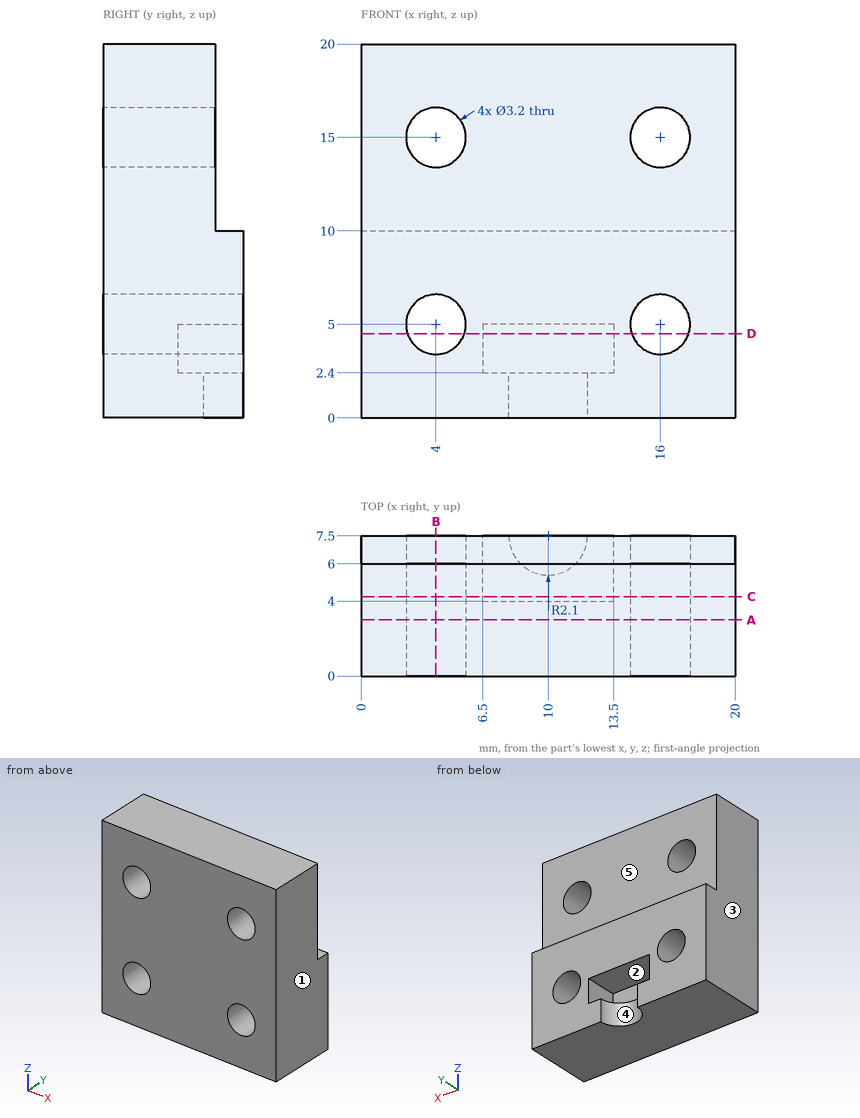
Here's the drawing with two shaded views (mm, measured from the low corner). I have some questions. A direction names the side the tool comes from. Coordinates: 2 decimals unless noted, no trailing zeros. Write each loop counter-clockwise with the first axis right and the second up, starting at its lowest first coordinate (ties: lowest second). Pieces come first, ordered by that corner, then holes. Notation, with made-up numbers: M 57.25,33.5 L 116.25,33.5 A32 ccw 116.25,59.5 Z; hole C 74,15.25 d2. An arc over 180 degrees is marked long. Answer as CSV lines item,"result". Start each with the question number.
1) For P1, Ø5, axis at x = 5.5, z = 14, coming from the +Y side; P2, Ø1.2, axis at x = 9.5, y = 7, coming from the +Z side; P3, Ø0.8, axis at x = 11.5, z = 3.5, coming from the +Y side, each with a flat end and sliding along its axis, tell me the tip position at first contact or that it passes through.
2) For the marked faces 1 and 2, which set-ups out of +Z, -Z, +X, -X, +Y, -Y let a thin tool reach every point of the face, with its end or its side?
3) We'd pull the mould along X, two halves only. Please class the marked faces 3, 4 and 5: +X half, -X half, draft (parallel to the pull), parting line (faces both ways), or undercut.
4) Please list where these lines run through material, in increasing order: line 1 (Z direction, x = 16, y = 2.75); line 2 (X direction, y = 3.4, z = 15); line 3 (X direction, y = 1, z = 15.5). Write a range as from..to.
5) I want a section at A-A, the plane y = 3. Please give me the cut outline in (x, z).
6) I want a section at D-D, the plane z = 4.5. Please give me the cut outline in (x, y), and give its area (3 significant figures).
7) I want a section at B-B, the plane x = 4. Please give me the cut outline in (y, z).
8) I want a section at C-C, the plane y = 4.25. Please give me the cut outline in (x, z), and give its area (3 significant figures).
Data:
1,P1,"stops at y = 6"
1,P2,"stops at z = 10"
1,P3,"stops at y = 4"
2,face 1,"+Z, -Z, +X, +Y, -Y"
2,face 2,"+Y"
3,face 3,"-X half"
3,face 4,"undercut"
3,face 5,"draft"
4,line 1,"z = 0..3.4, 6.6..13.4, 16.6..20"
4,line 2,"x = 0..2.4, 5.6..14.4, 17.6..20"
4,line 3,"x = 0..2.48, 5.52..14.48, 17.52..20"
5,outline,"M 0,0 L 20,0 L 20,20 L 0,20 Z; hole C 4,5 d3.2; hole C 4,15 d3.2; hole C 16,5 d3.2; hole C 16,15 d3.2"
6,outline,"M 0,0 L 2.48,0 L 2.48,7.5 L 0,7.5 Z; M 5.52,0 L 14.48,0 L 14.48,7.5 L 13.5,7.5 L 13.5,4 L 6.5,4 L 6.5,7.5 L 5.52,7.5 Z; M 17.52,0 L 20,0 L 20,7.5 L 17.52,7.5 Z"
6,area,"79.9 mm^2"
7,outline,"M 0,0 L 7.5,0 L 7.5,3.4 L 0,3.4 Z; M 0,6.6 L 7.5,6.6 L 7.5,10 L 6,10 L 6,13.4 L 0,13.4 Z; M 0,16.6 L 6,16.6 L 6,20 L 0,20 Z"
8,outline,"M 0,0 L 20,0 L 20,20 L 0,20 Z; hole C 4,5 d3.2; hole C 4,15 d3.2; hole M 6.5,2.4 L 13.5,2.4 L 13.5,5 L 6.5,5 Z; hole C 16,5 d3.2; hole C 16,15 d3.2"
8,area,"350 mm^2"
